from build123d import *

# Parameters (mm, degrees)
F1_DEPTH = 38.1
F2_R     = 27.603374
F3_DEPTH = 63.5


with BuildPart() as f1:
    # F0 (on Front) → F1 (new body)
    with BuildSketch(Plane.XZ):
        Polygon((51.004349, 40.765317), (-9.801625, 64.553721), (-60.805975, 23.788404), (-51.004349, -40.765317), (9.801625, -64.553721), (60.805975, -23.788404), align=None)
    extrude(amount=F1_DEPTH)

    # F2 (on face) → F3 (join)
    with BuildSketch(Plane.XZ.offset(38.1)):
        Circle(F2_R)
    extrude(amount=F3_DEPTH)


solid = f1.part
Verification items for the finished model (mm, model axes). A direction names the side the tool comes from. Coordinates: 2 decimals unless noted, no trailing zeros. Order: outer loops, then holes, each group sorted by start corner. A loop starts at its lowest first (then second) coordinate and runs counter-clockwise, first axis right, second up. Notation, with made-up numbers: (68.5, 20.5) -> (81.5, 20.5) arc R12 ccw to (81.5, 37.5) -> close; hole circle Ø1 at (79, 75.5). An arc over 180 degrees is marked (long way). Use CSV: the item, a comma, the result in double quotes. Start each with the question number.
Q1. Thickness scan on line 1 along Y through (x, z) = (34.5, -32); line 2 along Z through (x, y) = (1, -86.5); line 3 along Z through (x, y) = (38, -7). Record the ranges inside material, lowest first.
Q2. Depth check by flat-ended pin: P1, Ø1, axis at x = -45.5, z = -33, coming from the +Y side; P2, Ø5, axis at y = -87, z = -11.5, coming from the +X side; P3, Ø8, axis at y = -21, z = -4.5, coming from the -X side; P4, Ø5, axis at x = 27.5, y = -11, coming from the -Z side. Enter the tip coordinate at first touch or a pass-through.
Q3. Section check B-B, the plane x = -4. Record the cut outline in (y, z).
Q4. Tool access check on faces 1 (the flat face through (-55.974, -18.783, -8.037)), 2 (the cylindrical face through (-5.984, -69.406, -26.947)). Record the directions out of +Z, -Z, +X, -X, +Y, -Y that give a thin tool (end or side, any length) a straight path to the whole face; none if there is none.
Q5. Section check D-D, the plane y = -64. Record the cut outline in (x, z).
Q6. Section check C-C, the plane z = 0. Record the cut outline in (x, y), and give its area (3 significant figures).
Q7. Section check A-A, the plane y = -19. Record the cut outline in (x, z), and give its area (3 significant figures).
Returned:
1,line 1,"y = -38.1 to 0"
1,line 2,"z = -27.59 to 27.59"
1,line 3,"z = -42.02 to 45.85"
2,P1,"stops at y = 0"
2,P2,"stops at x = 26.09"
2,P3,"stops at x = -57.12"
2,P4,"stops at z = -52.41"
3,outline,"(-101.6, -27.31) -> (-38.1, -27.31) -> (-38.1, -59.15) -> (0, -59.15) -> (0, 62.28) -> (-38.1, 62.28) -> (-38.1, 27.31) -> (-101.6, 27.31) -> close"
4,face 1,"-Z, -X, +Y, -Y"
4,face 2,"-Y"
5,outline,"circle Ø55.21 at (0, 0)"
6,outline,"(-57.19, -38.1) -> (-27.6, -38.1) -> (-27.6, -101.6) -> (27.6, -101.6) -> (27.6, -38.1) -> (57.19, -38.1) -> (57.19, 0) -> (-57.19, 0) -> close"
6,area,"7,860 mm^2"
7,outline,"(-60.81, 23.79) -> (-51, -40.77) -> (9.8, -64.55) -> (60.81, -23.79) -> (51, 40.77) -> (-9.8, 64.55) -> close"
7,area,"11,100 mm^2"
